```python
from build123d import *

# Parameters (mm, degrees)
SKETCH1_W           = 82.55
SKETCH1_H           = 62.23
SKETCH1_R           = 1.778
SKETCH1_W_2         = 33
SKETCH1_H_2         = 28
BOSS_EXTRUDE1_DEPTH = 1.5
SKETCH2_W           = 2.642806411
SKETCH2_H           = 11.945484976
BOSS_EXTRUDE2_DEPTH = 1
SKETCH3_W           = 7.043654848
SKETCH3_H           = 10.402717652
BOSS_EXTRUDE3_DEPTH = 2


with BuildPart() as part:
    # Sketch1 → Boss-Extrude1 (new body)
    with BuildSketch(Plane.XY):
        with Locations((41.275, 31.115)):
            Rectangle(SKETCH1_W, SKETCH1_H)
        with Locations((3.81, 58.42)):
            Circle(SKETCH1_R, mode=Mode.SUBTRACT)
        with Locations((78.74, 58.42)):
            Circle(SKETCH1_R, mode=Mode.SUBTRACT)
        with Locations((78.74, 3.81)):
            Circle(SKETCH1_R, mode=Mode.SUBTRACT)
        with Locations((3.81, 3.81)):
            Circle(SKETCH1_R, mode=Mode.SUBTRACT)
        with Locations((49.05, 31)):
            Rectangle(SKETCH1_W_2, SKETCH1_H_2, mode=Mode.SUBTRACT)
    extrude(amount=BOSS_EXTRUDE1_DEPTH)

    # Sketch2 → Boss-Extrude2 (add)
    with BuildSketch(Plane.XY.offset(1.5)):
        with Locations((3.321403206, 17.857601098)):
            Rectangle(SKETCH2_W, SKETCH2_H)
    extrude(amount=BOSS_EXTRUDE2_DEPTH)

    # Sketch3 → Boss-Extrude3 (add)
    with BuildSketch(Plane(origin=(0, 0, 0), x_dir=(-1, 0, 0), z_dir=(0, 0, -1))):
        with Locations((-7.521827424, 32.54095227)):
            Rectangle(SKETCH3_W, SKETCH3_H)
    extrude(amount=BOSS_EXTRUDE3_DEPTH)


solid = part.part
```
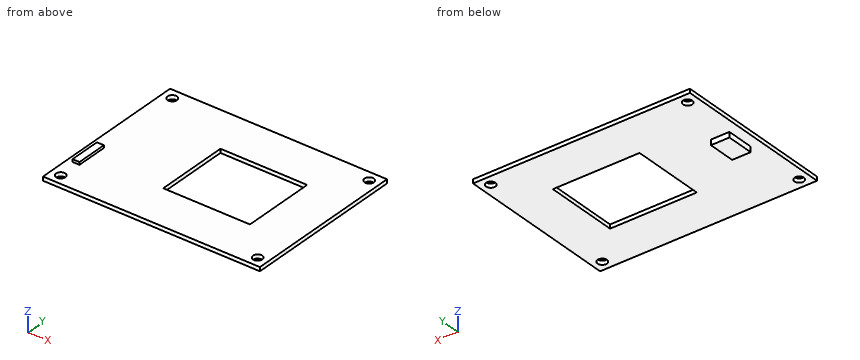
Design review of the part built by this model. Coordinates are the model's own, in mm. Coordinates: 2 decimals unless noted, no trailing zeros. Order: outer loops, then holes, each group sorted by start corner. A loop starts at its lowest first (then second) coordinate and runs counter-clockwise, first axis right, second up. Notation, with made-up numbers: (0.5, 22) -> (32.5, 22) arc R15 ccw to (32.5, 40) -> close; hole circle Ø2 at (62, -21.75). An arc over 180 degrees is marked (long way). One line per item, written item: value. Start each with the question number.
Q1. For probe 1 along X at (y, z) = (4, 1.2); probe 2 along Y at (x, z) = (78.74, 0.55); probe 3 along Y at (x, z) = (39, 1.1), list the stretches that pass through material, from the lowest coordinate up.
Q2. Take a section at C-C, the plane x = 78.74. State the section outline as (y, z) points, then the cut area to 3 significant figures.
Q3. Take a section at B-B, the plane x = 58.5. State the section outline as (y, z) points.
Q4. Take a section at D-D, the plane y = 3.81. State the section outline as (x, z) points, then the cut area to 3 significant figures.
Q5. Take a section at A-A, the plane y = 33. State the section outline as (x, z) points, then the cut area to 3 significant figures.
Q6. Insertion check: pin 1 Ø2 at (y, z) = (32.5, -1.5) entering from +X; pin 2 Ø10 at (x, y) = (23.5, 46) entering from +Z; pin 3 Ø0.8 at (x, z) = (3.5, 2) entering from -Y; pin 4 Ø1.5 at (x, y) = (64, 35) entering from -Z. Each pin has a flat end and moves straight along its axis. Give the tip position at first contact, or say it passes through.
Values follow:
1. probe 1: x = 0 to 2.04, 5.58 to 76.97, 80.51 to 82.55
1. probe 2: y = 0 to 2.03, 5.59 to 56.64, 60.2 to 62.23
1. probe 3: y = 0 to 17, 45 to 62.23
2. outline: (0, 0) -> (2.03, 0) -> (2.03, 1.5) -> (0, 1.5) -> close; (5.59, 0) -> (56.64, 0) -> (56.64, 1.5) -> (5.59, 1.5) -> close; (60.2, 0) -> (62.23, 0) -> (62.23, 1.5) -> (60.2, 1.5) -> close
2. area: 82.7 mm2
3. outline: (0, 0) -> (17, 0) -> (17, 1.5) -> (0, 1.5) -> close; (45, 0) -> (62.23, 0) -> (62.23, 1.5) -> (45, 1.5) -> close
4. outline: (0, 0) -> (2.03, 0) -> (2.03, 1.5) -> (0, 1.5) -> close; (5.59, 0) -> (76.96, 0) -> (76.96, 1.5) -> (5.59, 1.5) -> close; (80.52, 0) -> (82.55, 0) -> (82.55, 1.5) -> (80.52, 1.5) -> close
4. area: 113 mm2
5. outline: (0, 0) -> (4, 0) -> (4, -2) -> (11.04, -2) -> (11.04, 0) -> (32.55, 0) -> (32.55, 1.5) -> (0, 1.5) -> close; (65.55, 0) -> (82.55, 0) -> (82.55, 1.5) -> (65.55, 1.5) -> close
5. area: 88.4 mm2
6. pin 1: stops at x = 11.04
6. pin 2: stops at z = 1.5
6. pin 3: stops at y = 11.88
6. pin 4: passes through
